```python
from build123d import *

# Parameters (mm, degrees)
SKETCH1_W             = 80
SKETCH1_H             = 180
SKETCH1_R             = 8.5
BOSS_EXTRUDE1_DEPTH   = 5
SKETCH2_R             = 5.5
CUT_EXTRUDE1_DEPTH    = 30
SKETCH3_R             = 1.6
SKETCH3_R_2           = 2.5
CUT_EXTRUDE2_DEPTH    = 5
CUT_EXTRUDE3_DEPTH    = 10
BOSS_EXTRUDE2_DEPTH   = 5
FILLET1_R             = 2
FILLET2_R             = 5
SKETCH6_R             = 2.1
CUT_EXTRUDE4_DEPTH    = 5
SKETCH7_W             = 58.3648838
SKETCH7_H             = 19.178580611
BOSS_EXTRUDE3_DEPTH   = 5
SKETCH8_R             = 2.1
CUT_EXTRUDE5_DEPTH    = 5
SKETCH9_R             = 1.6
CUT_EXTRUDE6_DEPTH    = 5
SKETCH10_R            = 3
SKETCH10_R_2          = 1.6
BOSS_EXTRUDE4_DEPTH   = 5
BOSS_EXTRUDE4_2_DEPTH = 5
BOSS_EXTRUDE4_3_DEPTH = 5
BOSS_EXTRUDE4_4_DEPTH = 5
SKETCH11_R            = 5.5
BOSS_EXTRUDE5_DEPTH   = 5
FILLET3_R             = 3
CUT_EXTRUDE7_DEPTH    = 5
FILLET5_R             = 5


with BuildPart() as part:
    # Sketch1 → Boss-Extrude1 (new body)
    with BuildSketch(Plane.XY):
        with Locations((10, 166)):
            Rectangle(SKETCH1_W, SKETCH1_H)
        with Locations((20, 226)):
            Circle(SKETCH1_R, mode=Mode.SUBTRACT)
    extrude(amount=BOSS_EXTRUDE1_DEPTH)

    # Sketch2 → Cut-Extrude1 (cut)
    with BuildSketch(Plane.XY.offset(5)):
        with Locations((20, 151)):
            Circle(SKETCH2_R)
    extrude(amount=-CUT_EXTRUDE1_DEPTH, mode=Mode.SUBTRACT)

    # Sketch3 → Cut-Extrude2 (cut)
    with BuildSketch(Plane.XY.offset(5)):
        with Locations((0, 182)):
            Circle(SKETCH3_R)
        with Locations((25, 129.301270189)):
            Circle(SKETCH3_R)
        with Locations((-25.032859693, 102.533479235)):
            Circle(SKETCH3_R)
        with Locations((-15, 81)):
            Circle(SKETCH3_R_2)
        with Locations((15, 81)):
            Circle(SKETCH3_R_2)
        with Locations((24, 91)):
            Circle(SKETCH3_R_2)
        with Locations((-24, 91)):
            Circle(SKETCH3_R_2)
    extrude(amount=-CUT_EXTRUDE2_DEPTH, mode=Mode.SUBTRACT)

    # Sketch4 → Cut-Extrude3 (cut)
    with BuildSketch(Plane.XY.offset(5)):
        with BuildLine():
            Line((-30, 194.384776311), (10.807611845, 235.192388155))
            ThreePointArc((10.807611845, 235.192388155), (24.974884621, 238.010433923), (33, 226))
            ThreePointArc((33, 226), (32.888783198, 224.303159501), (32.557035742, 222.635352414))
            Line((32.557035742, 222.635352414), (22.786943589, 186.172872106))
            Line((22.786943589, 186.172872106), (30, 173.679491924))
            Line((30, 173.679491924), (30, 76))
            Line((30, 76), (50, 76))
            Line((50, 76), (50, 256))
            Line((50, 256), (-30, 256))
            Line((-30, 256), (-30, 194.384776311))
        make_face()
    extrude(amount=-CUT_EXTRUDE3_DEPTH, mode=Mode.SUBTRACT)

    # Sketch5 → Boss-Extrude2 (add)
    with BuildSketch(Plane.XY.offset(5)):
        with BuildLine():
            Line((-30, 169.384776311), (-30, 194.384776311))
            Line((-30, 194.384776311), (-46.535533906, 177.849242405))
            ThreePointArc((-46.535533906, 177.849242405), (-47.619397663, 176.227125661), (-48, 174.313708499))
            Line((-48, 174.313708499), (-48, 96.071067812))
            ThreePointArc((-48, 96.071067812), (-47.619397663, 94.15765065), (-46.535533906, 92.535533906))
            Line((-46.535533906, 92.535533906), (-30, 76))
            Line((-30, 76), (-30, 101))
            ThreePointArc((-30, 101), (-35, 96), (-40, 101))
            Line((-40, 101), (-40, 131.707106781))
            Line((-40, 131.707106781), (-30, 121.707106781))
            Line((-30, 121.707106781), (-30, 138.67766953))
            Line((-30, 138.67766953), (-40, 148.67766953))
            Line((-40, 148.67766953), (-40, 169.384776311))
            ThreePointArc((-40, 169.384776311), (-35, 174.384776311), (-30, 169.384776311))
        make_face()
    extrude(amount=-BOSS_EXTRUDE2_DEPTH)

    # Fillet1
    fillet1_edges = [part.edges().sort_by_distance(p)[0] for p in [
        (-30, 121.707106781, 2.5),
        (-40, 131.707106781, 2.5),
        (-40, 148.67766953, 2.5),
        (-30, 138.67766953, 2.5),
    ]]
    fillet(fillet1_edges, radius=FILLET1_R)

    # Fillet2
    fillet2_edges = [part.edges().sort_by_distance(p)[0] for p in [
        (30, 173.679491924, 2.5),
        (22.786943589, 186.172872106, 2.5),
    ]]
    fillet(fillet2_edges, radius=FILLET2_R)

    # Sketch6 → Cut-Extrude4 (cut)
    with BuildSketch(Plane.XY.offset(5)):
        with Locations((15.982125076, 183.959163508)):
            Circle(SKETCH6_R)
    extrude(amount=-CUT_EXTRUDE4_DEPTH, mode=Mode.SUBTRACT)

    # Sketch7 → Boss-Extrude3 (add)
    with BuildSketch(Plane(origin=(0, 0, 0), x_dir=(-1, 0, 0), z_dir=(0, 0, -1))):
        with Locations((-0.8175581, 85.589290306)):
            Rectangle(SKETCH7_W, SKETCH7_H)
    extrude(amount=-BOSS_EXTRUDE3_DEPTH)

    # Sketch8 → Cut-Extrude5 (cut)
    with BuildSketch(Plane(origin=(0, 0, 0), x_dir=(-1, 0, 0), z_dir=(0, 0, -1))):
        with Locations((24, 81)):
            Circle(SKETCH8_R)
        with Locations((-24, 81)):
            Circle(SKETCH8_R)
    extrude(amount=-CUT_EXTRUDE5_DEPTH, mode=Mode.SUBTRACT)

    # Sketch9 → Cut-Extrude6 (cut)
    with BuildSketch(Plane(origin=(0, 0, 0), x_dir=(-1, 0, 0), z_dir=(0, 0, -1))):
        with Locations((-26, 176)):
            Circle(SKETCH9_R)
        with Locations((32, 176)):
            Circle(SKETCH9_R)
        with Locations((-26, 90)):
            Circle(SKETCH9_R)
        with Locations((32, 90)):
            Circle(SKETCH9_R)
    extrude(amount=-CUT_EXTRUDE6_DEPTH, mode=Mode.SUBTRACT)



with BuildPart() as body_2:
    # Sketch10 → Boss-Extrude4 (new body)
    with BuildSketch(Plane(origin=(0, 0, 0), x_dir=(-1, 0, 0), z_dir=(0, 0, -1))):
        with Locations((-34, 176)):
            Circle(SKETCH10_R)
        with Locations((-34, 176)):
            Circle(SKETCH10_R_2, mode=Mode.SUBTRACT)
    extrude(amount=-BOSS_EXTRUDE4_DEPTH)


with BuildPart() as body_3:
    # Sketch10 → Boss-Extrude4 2 (new body)
    with BuildSketch(Plane(origin=(0, 0, 0), x_dir=(-1, 0, 0), z_dir=(0, 0, -1))):
        with Locations((-34, 101)):
            Circle(SKETCH10_R)
        with Locations((-34, 101)):
            Circle(SKETCH10_R_2, mode=Mode.SUBTRACT)
    extrude(amount=-BOSS_EXTRUDE4_2_DEPTH)


with BuildPart() as body_4:
    # Sketch10 → Boss-Extrude4 3 (new body)
    with BuildSketch(Plane(origin=(0, 0, 0), x_dir=(-1, 0, 0), z_dir=(0, 0, -1))):
        with Locations((53, 176)):
            Circle(SKETCH10_R)
        with Locations((53, 176)):
            Circle(SKETCH10_R_2, mode=Mode.SUBTRACT)
    extrude(amount=-BOSS_EXTRUDE4_3_DEPTH)


with BuildPart() as body_5:
    # Sketch10 → Boss-Extrude4 4 (new body)
    with BuildSketch(Plane(origin=(0, 0, 0), x_dir=(-1, 0, 0), z_dir=(0, 0, -1))):
        with Locations((53, 101)):
            Circle(SKETCH10_R)
        with Locations((53, 101)):
            Circle(SKETCH10_R_2, mode=Mode.SUBTRACT)
    extrude(amount=-BOSS_EXTRUDE4_4_DEPTH)


with BuildPart() as part_1:
    add(part.part)

    add(body_2.part)  # Boss-Extrude5 merges body 2

    add(body_3.part)  # Boss-Extrude5 merges body 3

    add(body_4.part)  # Boss-Extrude5 merges body 4

    add(body_5.part)  # Boss-Extrude5 merges body 5
    # Sketch11 → Boss-Extrude5 (add)
    with BuildSketch(Plane(origin=(0, 0, 0), x_dir=(-1, 0, 0), z_dir=(0, 0, -1))):
        with Locations((-20, 151)):
            Circle(SKETCH11_R)
        with BuildLine():
            Line((30, 120.878679656), (30, 101))
            ThreePointArc((30, 101), (35, 96), (40, 101))
            Line((40, 101), (40, 126.878679656))
            ThreePointArc((40, 126.878679656), (38.765366865, 128.726438721), (36.585786438, 128.292893219))
            Line((36.585786438, 128.292893219), (30.585786438, 122.292893219))
            ThreePointArc((30.585786438, 122.292893219), (30.152240935, 121.644046521), (30, 120.878679656))
        make_face()
        with BuildLine():
            Line((40, 169.384776311), (40, 149.506096654))
            ThreePointArc((40, 149.506096654), (39.847759065, 148.74072979), (39.414213562, 148.091883092))
            Line((39.414213562, 148.091883092), (33.414213562, 142.091883092))
            ThreePointArc((33.414213562, 142.091883092), (31.234633135, 141.658337589), (30, 143.506096654))
            Line((30, 143.506096654), (30, 169.384776311))
            ThreePointArc((30, 169.384776311), (35, 174.384776311), (40, 169.384776311))
        make_face()
        with BuildLine():
            Line((53.561989138, 178.946891279), (43.523484359, 180.861291952))
            Line((43.523484359, 180.861291952), (46.535533906, 177.849242405))
            ThreePointArc((46.535533906, 177.849242405), (47.619397663, 176.227125661), (48, 174.313708499))
            Line((48, 174.313708499), (48, 166.595931299))
            Line((48, 166.595931299), (55.144920857, 173.902545705))
            ThreePointArc((55.144920857, 173.902545705), (50.137624065, 175.101777308), (53.561989138, 178.946891279))
        make_face()
        with BuildLine():
            Line((55.144920857, 103.097454295), (48, 110.404068701))
            Line((48, 110.404068701), (48, 96.071067812))
            ThreePointArc((48, 96.071067812), (47.619397663, 94.15765065), (46.535533906, 92.535533906))
            Line((46.535533906, 92.535533906), (54.774786308, 98.581295065))
            ThreePointArc((54.774786308, 98.581295065), (50.010025149, 101.24505181), (55.144920857, 103.097454295))
        make_face()
        with BuildLine():
            Line((-34.922393234, 178.854678742), (-25.198007946, 181.99678614))
            Line((-25.198007946, 181.99678614), (-29.330127019, 174.839745962))
            ThreePointArc((-29.330127019, 174.839745962), (-29.829629131, 173.633841188), (-30, 172.339745962))
            Line((-30, 172.339745962), (-30, 166.12900673))
            Line((-30, 166.12900673), (-36.350455148, 174.135768095))
            ThreePointArc((-36.350455148, 174.135768095), (-31.128604249, 175.1310429), (-34.922393234, 178.854678742))
        make_face()
        with BuildLine():
            Line((-36.350455148, 102.864231905), (-30, 110.87099327))
            Line((-30, 110.87099327), (-30, 91.12900673))
            Line((-30, 91.12900673), (-36.350455148, 99.135768095))
            ThreePointArc((-36.350455148, 99.135768095), (-31, 101), (-36.350455148, 102.864231905))
        make_face()
    extrude(amount=-BOSS_EXTRUDE5_DEPTH)

    # Fillet3
    fillet3_edges = [part_1.edges().sort_by_distance(p)[0] for p in [
        (-46.535533906, 92.535533906, 2.5),
        (-48, 166.595931299, 2.5),
        (-43.523484359, 180.861291952, 2.5),
        (-48, 110.404068701, 2.5),
        (25.198007946, 181.99678614, 2.5),
        (30, 166.12900673, 2.5),
        (30, 110.87099327, 2.5),
        (30, 91.12900673, 2.5),
    ]]
    fillet(fillet3_edges, radius=FILLET3_R)

    # Sketch12 → Cut-Extrude7 (cut)
    with BuildSketch(Plane(origin=(0, 0, 0), x_dir=(-1, 0, 0), z_dir=(0, 0, -1))):
        with BuildLine():
            Line((-18.698443457, 209.551414937), (-13.933365214, 191.767900833))
            Line((-13.933365214, 191.767900833), (23.002512143, 187.240128544))
            Line((23.002512143, 187.240128544), (-6.405885751, 216.648526438))
            ThreePointArc((-6.405885751, 216.648526438), (-11.75, 211.710580838), (-18.698443457, 209.551414937))
        make_face()
        Polygon((-13.933365214, 175.648133085), (-13.933365214, 120.954454576), (36, 169.527068053), align=None)
        Polygon((36, 152.786143643), (11.352419227, 128.810242782), (36, 107.935659547), align=None)
        Polygon((4.150846245, 121.804922404), (-13.933365214, 104.213530166), (-13.933365214, 86), (17.032859693, 86), (17.032859693, 110.894859285), align=None)
    extrude(amount=-CUT_EXTRUDE7_DEPTH, mode=Mode.SUBTRACT)

    # Fillet5
    fillet5_edges = [part_1.edges().sort_by_distance(p)[0] for p in [
        (18.698443457, 209.551414937, 2.5),
        (6.405885751, 216.648526438, 2.5),
        (-23.002512143, 187.240128544, 2.5),
        (13.933365214, 191.767900833, 2.5),
        (-17.032859693, 86, 2.5),
        (13.933365214, 86, 2.5),
        (13.933365214, 104.213530166, 2.5),
        (-4.150846245, 121.804922404, 2.5),
        (-17.032859693, 110.894859285, 2.5),
        (13.933365214, 175.648133085, 2.5),
        (-36, 169.527068053, 2.5),
        (13.933365214, 120.954454576, 2.5),
        (-36, 152.786143643, 2.5),
        (-36, 107.935659547, 2.5),
        (-11.352419227, 128.810242782, 2.5),
    ]]
    fillet(fillet5_edges, radius=FILLET5_R)


solid = part_1.part
```
Input: part model. Units: mm. Frame: model coordinates. A direction names the side the tool comes from. Give positions to 0.01 mm unless a question says otherwise; leave off trailing zeros. Order: outer loops, then holes, each group sorted by start corner. A loop starts at its lowest first (then second) coordinate and runs counter-clockwise, first axis right, second up.
1. Section D-D on x = -32. Return the cut outline in (y, z), and give its area (3 significant figures).
Derived:
outline: (78, 0) - (88.4, 0) - (88.4, 5) - (78, 5) - close; (91.6, 0) - (113.82, 0) - (113.82, 5) - (91.6, 5) - close; (145.85, 0) - (174.4, 0) - (174.4, 5) - (145.85, 5) - close; (177.6, 0) - (192.38, 0) - (192.38, 5) - (177.6, 5) - close
area: 380 mm2
2. Reachability of faces 1 (the flat face through (-52.04, 106.27, 2.46)), 2 (the cylindrical face through (13.288, 192.574, 2.535)), 3 (the flat face through (30, 139, 3)) from +Z, -Z, +X, -X, +Y, -Y: full face, straight path, thin tool, end or side. Return the list, or none.
Derived:
face 1: +Z, -Z, -X
face 2: +Z, -Z
face 3: +Z, -Z, +X
3. Section A-A on y = 81. Return the cut outline in (x, z), and give its area (3 significant figures).
Derived:
outline: (-35, 0) - (-26.1, 0) - (-26.1, 5) - (-35, 5) - close; (-21.9, 0) - (21.9, 0) - (21.9, 5) - (-21.9, 5) - close; (26.1, 0) - (30, 0) - (30, 5) - (26.1, 5) - close
area: 283 mm2
4. Section B-B on x = 20. Return the cut outline in (y, z).
Derived:
outline: (76, 0) - (217.5, 0) - (217.5, 5) - (76, 5) - close; (234.5, 0) - (239, 0) - (239, 5) - (234.5, 5) - close
5. Mould query, pull axis Y, two halves, no side actions, for faces 4 (the flat face through (30, 83, 3)), 5 (the flat face through (-38, 84, 3)), 6 (the flat face through (13.933, 152, 2)). Classes: released by +Y, released by -Y, zero draft, split by the parting line, or undercut.
Derived:
face 4: zero draft
face 5: released by -Y
face 6: undercut
6. Pin query (flat end, axial travel): pin 1 (5 mm diameter, centred on x = -25.5, y = 170, fed in from +Z); pin 2 (1.5 mm diameter, centred on y = 104.5, z = 4, fed in from +X); pin 3 (2.5 mm diameter, centred on y = 145.5, z = 1.5, fed in from -X); pin 4 (2.5 mm diameter, centred on y = 135.5, z = 1.5, fed in from +X). Return the tip coordinate at first contact, or that it passes through.
Derived:
pin 1: stops at z = 5
pin 2: stops at x = 35.65
pin 3: stops at x = -48
pin 4: stops at x = 30
7. Section C-C on y = 209. Return the cut outline in (x, z), and give its area (3 significant figures).
Derived:
outline: (-15.38, 0) - (-1.24, 0) - (-1.24, 5) - (-15.38, 5) - close; (16.4, 0) - (28.9, 0) - (28.9, 5) - (16.4, 5) - close
area: 133 mm2
8. Material intervals for L1, parallel to X at y = 176, z = 2.65; L2, parallel to Y at x = 20, z = 1.75; L3, parallel to X at y = 132, z = 0.95, sorted ascending.
Derived:
L1: x = -56 to -54.6, -51.4 to -33.6, -30.4 to 24.4, 27.6 to 32.4, 35.6 to 37
L2: y = 76 to 217.5, 234.5 to 239
L3: x = -48 to -36, -14.74 to 2.58, 13.87 to 30
